Check sheet for the modelled part. Datum: model origin and axes. Units: mm. Face numbers are marked on the shaded views. Round coordinates to 2 decimals unless told otherwise and drop trailing zeros. Order: outer loops, then holes, each group sorted by start corner. A loop starts at its lowest first (then second) coordinate and runs counter-clockwise, first axis right, second up. Notation, with made-up numbers: (-37.75, -25.5) -> (-4.75, -25.5) arc R32 cw to (-4.75, 7.5) -> close; hole circle Ø4 at (71.5, 67). An arc over 180 degrees is marked (long way). Use CSV: the item, a comma, the result in double quotes.
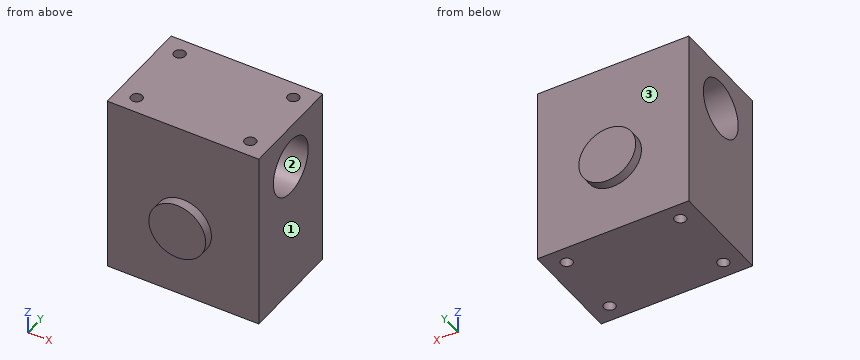
Autodesk Inventor part; units mm, degrees
ref_plane "YZ Plane" through (0, 0, 0) normal (1, 0, 0) x (0, 1, 0)
ref_plane "XZ Plane" through (0, 0, 0) normal (0, 1, 0) x (-1, 0, 0)
ref_plane "XY Plane" through (0, 0, 0) normal (0, 0, 1) x (1, 0, 0)
sketch "草圖1" plane through (0, 0, 0) normal (0, 0, 1) x (1, 0, 0)
  line L0 (-40, 27.5) -> (40, 27.5)
  line L1 (40, 27.5) -> (40, -27.5)
  line L2 (40, -27.5) -> (-40, -27.5)
  line L3 (-40, -27.5) -> (-40, 27.5)
  line L4 (-40, 27.5) -> (40, -27.5) construction
  line L5 (40, 27.5) -> (-40, -27.5) construction
  circle A0 centre (0, 0) radius 18.5
  circle A1 centre (0, -18.5) radius 30
  circle A2 centre (-30, -18.5) radius 3
  circle A3 centre (30, -18.5) radius 3
  circle A4 centre (0, 18.5) radius 30
  circle A5 centre (-30, 18.5) radius 3
  circle A6 centre (30, 18.5) radius 3
  dimension "d0" = 80
  dimension "d1" = 55
  dimension "d4" = 37
  dimension "d5" = 60
  dimension "d6" = 6
  dimension "d7" = 6
  dimension "d8" = 60
  dimension "d9" = 6
  dimension "d10" = 6
extrude "擠出1" add sketch "草圖1" along normal blind 95 contours L0 A4 A5 A1 A2 L2 L3 | L0 A4 A6 A1 A0 A5 | L0 L1 L2 A1 A3 A4 A6 | A1 A2 A4 A0 A3 L2 | A1 A0 A4 | A4 A0 A1 | A1 A0 A4 | A0 A1 | A4 A0
sketch "草圖2" plane through (-40, -27.5, 0) normal (-1, 0, 0) x (0, 0, 1)
  line L0 (95, 0) -> (95, 55)
  circle A0 centre (95, 0) radius 27.5
  circle A1 centre (95, 27.5) radius 23
  circle A2 centre (72, 27.5) radius 15
  point P0 (0, 27.5)
  dimension "d11" = 46
  dimension "d12" = 30
extrude "擠出2" cut sketch "草圖2" along normal through all both and the other way through all contours A2 A0 A1 | A1 A0 A2 | A0 A1 A2 | A0 A2 A1 picked at (73.0639, 14.4683) picked at (77.5879, 17.5315) picked at (79.9817, 30.5353) picked at (67.7059, 31.4722)
sketch "草圖3" plane through (-40, 27.5, 0) normal (0, 1, 0) x (1, 0, 0)
  circle A0 centre (40, 0) radius 40
  circle A1 centre (40, -40) radius 15
  dimension "d15" = 80
  dimension "d16" = 30
extrude "擠出3" add sketch "草圖3" along normal blind 5 and the other way blind 60 contours A1 A0 | A0 A1 picked at (35.277, -35.2849) picked at (34.8016, -43.9729)
properties part number "MotorPart1"
Q1. Sectioned sample at B-B, the plane y = 0. Enter the section's corners in (x, z), then the cut area to 3 significant figures.
Result sheet:
outline,"(-40, 0) -> (40, 0) -> (40, 57) -> (-40, 57) -> close; (-40, 87) -> (40, 87) -> (40, 95) -> (-40, 95) -> close"
area,"5,200 mm^2"
Q2. Go/stop test with flat-tipped pins: pin 1 (5 mm diameter, centred on x = 25, z = 43.5, fed in from -Y); pin 2 (1.5 mm diameter, centred on x = 29, z = 27.5, fed in from +Y). Record where each tip stops, or that it passes through.
Result sheet:
pin 1,"stops at y = -27.5"
pin 2,"stops at y = 27.5"
Q3. Scan lines: L1, parallel to X at y = -18.5, z = 32.5; L2, parallel to Y at x = -30, z = 43; L3, parallel to Y at x = -30, z = 72. Record each from-to range of solid material in increasing order.
Result sheet:
L1,"x = -40 to -33, -27 to 27, 33 to 40"
L2,"y = -27.5 to -21.5, -15.5 to 15.5, 21.5 to 27.5"
L3,"y = -27.5 to -21.5, -15.5 to -15, 15 to 15.5, 21.5 to 27.5"
Q4. Mould release check, pull along Y, two halves, no side actions. Record for the marked faces 1, 2 and 3: pulls with the +Y half, pulls with the -Y half, needs draft (parallel to the pull), parting line crosses it, or undercut.
Result sheet:
face 1,"needs draft"
face 2,"undercut"
face 3,"pulls with the +Y half"
Q5. Sectioned sample at A-A, the plane x = -30. Enter the section's corners in (y, z).
Result sheet:
outline,"(-27.5, 0) -> (-21.5, 0) -> (-21.5, 95) -> (-27.5, 95) -> close; (-15.5, 0) -> (15.5, 0) -> (15.5, 95) -> (-15.5, 95) -> close; (21.5, 0) -> (27.5, 0) -> (27.5, 95) -> (21.5, 95) -> close; hole circle Ø30 at (0, 72)"
Q6. Sectioned sample at D-D, the plane y = 18.5. Enter the section's corners in (x, z).
Result sheet:
outline,"(-40, 0) -> (-33, 0) -> (-33, 95) -> (-40, 95) -> close; (-27, 0) -> (27, 0) -> (27, 95) -> (-27, 95) -> close; (33, 0) -> (40, 0) -> (40, 95) -> (33, 95) -> close"
Q7. Sectioned sample at C-C, the plane z = 40. Enter the section's corners in (x, y).
Result sheet:
outline,"(-40, -27.5) -> (-15, -27.5) -> (-15, -32.5) -> (15, -32.5) -> (15, -27.5) -> (40, -27.5) -> (40, 27.5) -> (15, 27.5) -> (15, 32.5) -> (-15, 32.5) -> (-15, 27.5) -> (-40, 27.5) -> close; hole circle Ø6 at (-30, -18.5); hole circle Ø6 at (-30, 18.5); hole circle Ø6 at (30, -18.5); hole circle Ø6 at (30, 18.5)"
